Verification items for the finished model (mm, model axes). Face numbers are marked on the shaded views. A direction names the side the tool comes from. Coordinates: 2 decimals unless noted, no trailing zeros. Order: outer loops, then holes, each group sorted by start corner. A loop starts at its lowest first (then second) coordinate and runs counter-clockwise, first axis right, second up. Notation, with made-up numbers: M 67,18 L 88,18 A22 cw 88,45 Z; hole C 73,-5.75 d4. An arc over 180 degrees is marked long. Return JSON: item names as keys, results as strings. Group by question number.
1. Material ranges on line 1 along X through (y, z) = (7.5, 2.5); line 2 along Z through (x, y) = (-12, 6); line 3 along Y through (x, z) = (4.5, 13.5), recorded low to high.
2. Section check A-A, the plane y = 4.75. Record the cut outline in (x, z), plus the area to 3 significant figures.
3. Mould release check, pull along X, two halves, no side actions. Record for the marked faces 5, 6 and 7: +X half, -X half, draft (parallel to the pull), parting line (faces both ways), or undercut.
4. Gauge pin test, flat ends, axial feed: pin 1 (5 mm diameter, centred on y = 5, z = 9.5, fed in from +X); pin 2 (1.3 mm diameter, centred on x = -9, y = 4.5, fed in from +Z); pin 3 (5 mm diameter, centred on x = 10.5, y = 4.5, fed in from +Z). Record the tip position at first contact, or that the pin passes through.
5. Section check D-D, the plane z = -3.5. Record the cut outline in (x, y).
6. Section check B-B, the plane z = 9. Record the cut outline in (x, y), plus the area to 3 significant figures.
7. Set-up check for the marked faces 1, 2, 3 and 4: record each of +Z, -Z, +X, -X, +Y, -Y from which the full face is reachable in a straight line by a thin tool's end or side.
8. Section check C-C, the plane x = -6. Record the cut outline in (y, z).
```python
from build123d import *

# Parameters (mm, degrees)
SKETCH1_W          = 50
SKETCH1_H          = 40
BOARD_DEPTH        = 1.6
OPAMP_DIP8_1_START = 1.6
SKETCH2_W          = 10.2
SKETCH2_H          = 7.6
OPAMP_DIP8_1_DEPTH = 4.5
OPAMP_DIP8_2_START = 1.6
SKETCH3_W          = 10.2
SKETCH3_H          = 7.6
OPAMP_DIP8_2_DEPTH = 4.5
LED_DRIVER_START   = 1.6
SKETCH4_W          = 8
SKETCH4_H          = 12
LED_DRIVER_DEPTH   = 6
HEADER_START       = 1.6
SKETCH5_W          = 2.5
SKETCH5_H          = 15
HEADER_DEPTH       = 8.5


with BuildPart() as part:
    # Sketch1 → Board (new body)
    with BuildSketch(Plane(origin=(0, 0, 0), x_dir=(1, 0, 0), z_dir=(0, 1, 0))):
        Rectangle(SKETCH1_W, SKETCH1_H)
    extrude(amount=BOARD_DEPTH)

    # Sketch2 → OpAmp_DIP8_1 (add)
    with BuildSketch(Plane(origin=(0, 0, 0), x_dir=(1, 0, 0), z_dir=(0, 1, 0)).offset(OPAMP_DIP8_1_START)):
        with Locations((-10, 8)):
            Rectangle(SKETCH2_W, SKETCH2_H)
    extrude(amount=OPAMP_DIP8_1_DEPTH)

    # Sketch3 → OpAmp_DIP8_2 (add)
    with BuildSketch(Plane(origin=(0, 0, 0), x_dir=(1, 0, 0), z_dir=(0, 1, 0)).offset(OPAMP_DIP8_2_START)):
        with Locations((-10, -8)):
            Rectangle(SKETCH3_W, SKETCH3_H)
    extrude(amount=OPAMP_DIP8_2_DEPTH)

    # Sketch4 → LED_Driver (add)
    with BuildSketch(Plane(origin=(0, 0, 0), x_dir=(1, 0, 0), z_dir=(0, 1, 0)).offset(LED_DRIVER_START)):
        with Locations((10, 0)):
            Rectangle(SKETCH4_W, SKETCH4_H)
    extrude(amount=LED_DRIVER_DEPTH)

    # Sketch5 → Header (add)
    with BuildSketch(Plane(origin=(0, 0, 0), x_dir=(1, 0, 0), z_dir=(0, 1, 0)).offset(HEADER_START)):
        with Locations((20, 0)):
            Rectangle(SKETCH5_W, SKETCH5_H)
    extrude(amount=HEADER_DEPTH)


solid = part.part
```
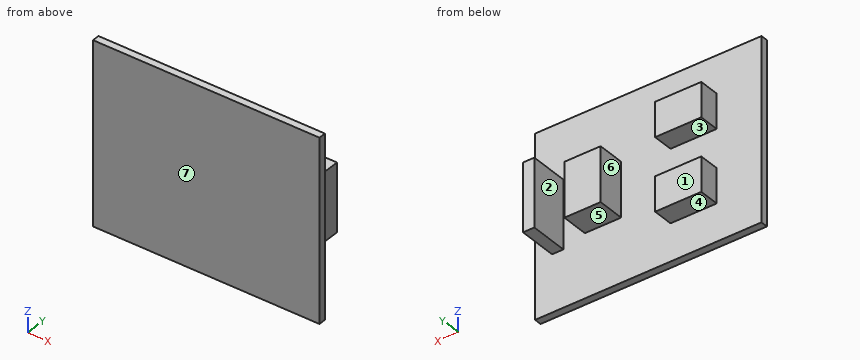
Answers follow:
{
 "1": {"line 1": "6 to 14, 18.75 to 21.25", "line 2": "-11.8 to -4.2, 4.2 to 11.8", "line 3": "0 to 1.6"},
 "2": {"outline": "M -15.1,-11.8 L -4.9,-11.8 L -4.9,-4.2 L -15.1,-4.2 Z; M -15.1,4.2 L -4.9,4.2 L -4.9,11.8 L -15.1,11.8 Z; M 6,-6 L 14,-6 L 14,6 L 6,6 Z; M 18.75,-7.5 L 21.25,-7.5 L 21.25,7.5 L 18.75,7.5 Z", "area": "289 mm^2"},
 "3": {"face 5": "undercut", "face 6": "undercut", "face 7": "draft"},
 "4": {"pin 1": "x = 21.25", "pin 2": "z = 11.8", "pin 3": "z = 6"},
 "5": {"outline": "M -25,0 L 25,0 L 25,1.6 L 21.25,1.6 L 21.25,10.1 L 18.75,10.1 L 18.75,1.6 L 14,1.6 L 14,7.6 L 6,7.6 L 6,1.6 L -25,1.6 Z"},
 "6": {"outline": "M -25,0 L 25,0 L 25,1.6 L -4.9,1.6 L -4.9,6.1 L -15.1,6.1 L -15.1,1.6 L -25,1.6 Z", "area": "126 mm^2"},
 "7": {"face 1": "+Z, -Z, -X, +Y", "face 2": "+Z, -Z, +Y", "face 3": "-X, +Y", "face 4": "-Z, +X, -X, +Y"},
 "8": {"outline": "M 0,-20 L 1.6,-20 L 1.6,-11.8 L 6.1,-11.8 L 6.1,-4.2 L 1.6,-4.2 L 1.6,4.2 L 6.1,4.2 L 6.1,11.8 L 1.6,11.8 L 1.6,20 L 0,20 Z"}
}
